Source: CAD feature listing. Evaluate the final solid. Frame: model axes, mm. Give positions to 0.01 mm unless a question says otherwise; leave off trailing zeros. Loops run counter-clockwise (first coordinate to the right, second up) from the corner with the lowest first, then second, coordinate; pieces in that order, holes last.
Autodesk Inventor part; units mm, degrees
ref_plane "YZ Plane" through (0, 0, 0) normal (1, 0, 0) x (0, 1, 0)
ref_plane "XZ Plane" through (0, 0, 0) normal (0, 1, 0) x (-1, 0, 0)
ref_plane "XY Plane" through (0, 0, 0) normal (0, 0, 1) x (1, 0, 0)
sketch "Esquisse1" plane through (0, 0, 0) normal (0, 1, 0) x (-1, 0, 0)
  line L0 (81.9588, 98.0854) -> (-168.0412, 98.0854)
  line L1 (-168.0412, 98.0854) -> (-168.0412, -201.9146)
  line L2 (-168.0412, -201.9146) -> (81.9588, -201.9146)
  line L3 (81.9588, -201.9146) -> (81.9588, 98.0854)
  point P0 (0, 0)
  dimension "d0" = 300
  dimension "d1" = 250
extrude "Extrusion1" add sketch "Esquisse1" along normal blind 5
sketch "Sketch3" plane through (0, 5, 0) normal (0, 1, 0) x (1, 0, 0)
  line L0 (81.0412, -85.0854) -> (5.0412, -85.0854)
  line L1 (5.0412, -85.0854) -> (5.0412, -17.0854)
  line L2 (81.0412, -17.0854) -> (81.0412, -85.0854)
  line L3 (-81.9588, -98.0854) -> (168.0412, -98.0854)
  line L4 (168.0412, -98.0854) -> (168.0412, 201.9146)
  line L5 (17.0412, -17.0854) -> (17.0412, 40.9146)
  line L6 (17.0412, 40.9146) -> (69.0412, 40.9146)
  line L7 (69.0412, 40.9146) -> (69.0412, -17.0854)
  line L8 (5.0412, -17.0854) -> (17.0412, -17.0854)
  line L9 (69.0412, -17.0854) -> (81.0412, -17.0854)
  line L10 (81.0412, 188.9146) -> (5.0412, 188.9146)
  line L11 (5.0412, 188.9146) -> (5.0412, 120.9146)
  line L12 (81.0412, 120.9146) -> (81.0412, 188.9146)
  line L13 (168.0412, 201.9146) -> (-81.9588, 201.9146)
  line L14 (17.0412, 120.9146) -> (17.0412, 62.9146)
  line L15 (17.0412, 62.9146) -> (69.0412, 62.9146)
  line L16 (69.0412, 62.9146) -> (69.0412, 120.9146)
  line L17 (5.0412, 120.9146) -> (17.0412, 120.9146)
  line L18 (69.0412, 120.9146) -> (81.0412, 120.9146)
  circle A0 centre (85.0412, 51.9146) radius 1.5
  line L19 (-81.9588, 201.9146) -> (-81.9588, -98.0854)
  circle A1 centre (1.0412, 51.9146) radius 1.5
  point P0 (0, 0)
  dimension "d17" = 76
  dimension "d18" = 68
  dimension "d19" = 13
  dimension "d20" = 87
  dimension "d21" = 12
  dimension "d22" = 12
  dimension "d23" = 58
  dimension "d24" = 68
  dimension "d25" = 52
  dimension "d26" = 13
  dimension "d27" = 76
  dimension "d28" = 68
  dimension "d29" = 87
  dimension "d30" = 12
  dimension "d31" = 12
  dimension "d32" = 58
  dimension "d33" = 52
  dimension "d34" = 68
  dimension "d39" = 3
  dimension "d53" = 83
  dimension "d54" = 150
  dimension "d58" = 3
  dimension "d59" = 83
  dimension "d60" = 150
extrude "Extrusion3" cut sketch "Sketch3" against normal through all contours L0 L1 L8 L5 L6 L7 L9 L2 | L12 L18 L16 L15 L14 L17 L11 L10 | A0 | A1
sketch "Sketch4" plane through (0, 5, 0) normal (0, 1, 0) x (1, 0, 0)
  circle A0 centre (1.0412, -89.0854) radius 1.5
  circle A1 centre (1.0412, -11.0854) radius 1.5
  circle A2 centre (85.0412, -89.0854) radius 1.5
  circle A3 centre (85.0412, -11.0854) radius 1.5
  circle A4 centre (1.0412, 114.9146) radius 1.5
  circle A5 centre (1.0412, 192.9146) radius 1.5
  circle A6 centre (85.0412, 192.9146) radius 1.5
  circle A7 centre (85.0412, 114.9146) radius 1.5
  point P0 (0, 0)
extrude "Extrusion4" cut sketch "Sketch4" against normal up to next
sketch "Esquisse5" plane through (0, 5, 0) normal (0, 1, 0) x (1, 0, 0)
  circle A0 centre (139.5412, -83.0854) radius 1.5
  circle A1 centre (133.0412, -83.0854) radius 1.5
  circle A2 centre (133.0412, 186.9146) radius 1.5
  circle A3 centre (139.5412, 186.9146) radius 1.5
  circle A4 centre (-41.9588, 186.9146) radius 1.5
  circle A5 centre (-48.4588, 186.9145) radius 1.4999
  circle A6 centre (-41.9588, -83.0854) radius 1.5
  circle A7 centre (85.0412, 192.9146) radius 1.5
  circle A8 centre (1.0412, 114.9146) radius 1.5
  circle A9 centre (85.0412, -89.0854) radius 1.5
  circle A10 centre (1.0412, -89.0854) radius 1.5
  circle A11 centre (1.0412, -11.0854) radius 1.5
  circle A12 centre (85.0412, -11.0854) radius 1.5
  circle A13 centre (1.0412, 192.9146) radius 1.5
  circle A14 centre (85.0412, 114.9146) radius 1.5
  line L0 (81.0412, -17.0854) -> (81.0412, -85.0854)
  line L1 (81.0412, -85.0854) -> (5.0412, -85.0854)
  line L2 (5.0412, -85.0854) -> (5.0412, -17.0854)
  line L3 (5.0412, -17.0854) -> (17.0412, -17.0854)
  line L4 (17.0412, -17.0854) -> (17.0412, 40.9146)
  line L5 (17.0412, 40.9146) -> (69.0412, 40.9146)
  line L6 (69.0412, 40.9146) -> (69.0412, -17.0854)
  line L7 (69.0412, -17.0854) -> (81.0412, -17.0854)
  circle A15 centre (85.0412, 51.9146) radius 1.5
  circle A16 centre (1.0412, 51.9146) radius 1.5
  line L8 (5.0412, 120.9146) -> (5.0412, 188.9146)
  line L9 (5.0412, 188.9146) -> (81.0412, 188.9146)
  line L10 (81.0412, 188.9146) -> (81.0412, 120.9146)
  line L11 (81.0412, 120.9146) -> (69.0412, 120.9146)
  line L12 (69.0412, 120.9146) -> (69.0412, 62.9146)
  line L13 (69.0412, 62.9146) -> (17.0412, 62.9146)
  line L14 (17.0412, 62.9146) -> (17.0412, 120.9146)
  line L15 (17.0412, 120.9146) -> (5.0412, 120.9146)
  line L16 (-81.9588, -98.0854) -> (168.0412, -98.0854)
  line L17 (168.0412, -98.0854) -> (168.0412, 201.9146)
  line L18 (168.0412, 201.9146) -> (-81.9588, 201.9146)
  line L19 (-81.9588, 201.9146) -> (-81.9588, -98.0854)
  circle A17 centre (-48.4588, -83.0854) radius 1.5
  point P0 (0, 0)
extrude "Extrusion5" cut sketch "Esquisse5" against normal up to next contours A0 | A1 | A2 | A3 | A4 | A5 | A6 | A17
sketch "Esquisse6" plane through (0, 0, 0) normal (0, -1, 0) x (1, 0, 0)
  circle A0 centre (139.0412, 63.0854) radius 1.5
  circle A1 centre (163.0412, 39.0854) radius 1.5
  circle A2 centre (139.0412, -142.9146) radius 1.5
  circle A3 centre (163.0412, -166.9146) radius 1.5
  line L0 (-81.9588, 98.0854) -> (168.0412, 98.0854)
  line L1 (168.0412, -201.9146) -> (-81.9588, -201.9146)
  line L2 (57.7912, 123.3914) -> (57.7912, -232.7016)
  line L3 (168.0412, 98.0854) -> (168.0412, -201.9146)
  circle A4 centre (-23.4588, 63.0854) radius 1.5
  circle A5 centre (-47.4588, 39.0854) radius 1.5
  circle A6 centre (-23.4588, -142.9146) radius 1.5
  circle A7 centre (-47.4588, -166.9146) radius 1.5
  point P0 (0, 0)
  dimension "d82" = 110.25
extrude "Extrusion6" cut sketch "Esquisse6" against normal up to next contours A0 | A1 | A2 | A3 | A4 | A5 | A6 | A7
sketch "Esquisse7" plane through (0, 5, 0) normal (0, 1, 0) x (1, 0, 0)
  circle A0 centre (152.0412, 161.9146) radius 1.5
  circle A1 centre (-65.9588, 51.9146) radius 1.5
  circle A2 centre (152.0412, 51.9146) radius 1.5
  circle A3 centre (152.0412, -58.0854) radius 1.5
  line L0 (-81.9588, 201.9146) -> (168.0412, 201.9146)
  line L1 (-81.9588, -98.0854) -> (-81.9588, 201.9146)
  line L2 (168.0412, -98.0854) -> (-81.9588, -98.0854)
  line L3 (168.0412, 201.9146) -> (168.0412, -98.0854)
  circle A4 centre (152.0412, 161.9146) radius 1.5
  circle A5 centre (-65.9588, 51.9146) radius 1.5
  circle A6 centre (152.0412, 51.9146) radius 1.5
  circle A7 centre (152.0412, -58.0854) radius 1.5
  line L4 (-81.9588, 201.9146) -> (168.0412, 201.9146)
  line L5 (-81.9588, -98.0854) -> (-81.9588, 201.9146)
  line L6 (168.0412, -98.0854) -> (-81.9588, -98.0854)
  line L7 (168.0412, 201.9146) -> (168.0412, -98.0854)
  circle A8 centre (152.0412, 161.9146) radius 1.5
  circle A9 centre (-65.9588, 51.9146) radius 1.5
  circle A10 centre (152.0412, 51.9146) radius 1.5
  circle A11 centre (152.0412, -58.0854) radius 1.5
  line L8 (-81.9588, 201.9146) -> (168.0412, 201.9146)
  line L9 (-81.9588, -98.0854) -> (-81.9588, 201.9146)
  line L10 (168.0412, -98.0854) -> (-81.9588, -98.0854)
  line L11 (168.0412, 201.9146) -> (168.0412, -98.0854)
  circle A12 centre (133.0412, -83.0854) radius 1.5
  circle A13 centre (-41.9588, 186.9146) radius 1.5
  circle A14 centre (133.0412, 186.9146) radius 1.5
  circle A15 centre (-48.4588, 186.9145) radius 1.4999
  circle A16 centre (139.5412, 186.9146) radius 1.5
  circle A17 centre (-41.9588, -83.0854) radius 1.5
  circle A18 centre (139.5412, -83.0854) radius 1.5
  circle A19 centre (-48.4588, -83.0854) radius 1.5
  circle A20 centre (85.0412, 192.9146) radius 1.5
  circle A21 centre (1.0412, 114.9146) radius 1.5
  circle A22 centre (85.0412, -89.0854) radius 1.5
  circle A23 centre (1.0412, -89.0854) radius 1.5
  circle A24 centre (1.0412, -11.0854) radius 1.5
  circle A25 centre (85.0412, -11.0854) radius 1.5
  circle A26 centre (1.0412, 192.9146) radius 1.5
  circle A27 centre (85.0412, 114.9146) radius 1.5
  line L12 (81.0412, -17.0854) -> (81.0412, -85.0854)
  line L13 (81.0412, -85.0854) -> (5.0412, -85.0854)
  line L14 (5.0412, -85.0854) -> (5.0412, -17.0854)
  line L15 (5.0412, -17.0854) -> (17.0412, -17.0854)
  line L16 (17.0412, -17.0854) -> (17.0412, 40.9146)
  line L17 (17.0412, 40.9146) -> (69.0412, 40.9146)
  line L18 (69.0412, 40.9146) -> (69.0412, -17.0854)
  line L19 (69.0412, -17.0854) -> (81.0412, -17.0854)
  circle A28 centre (85.0412, 51.9146) radius 1.5
  circle A29 centre (1.0412, 51.9146) radius 1.5
  line L20 (5.0412, 120.9146) -> (5.0412, 188.9146)
  line L21 (5.0412, 188.9146) -> (81.0412, 188.9146)
  line L22 (81.0412, 188.9146) -> (81.0412, 120.9146)
  line L23 (81.0412, 120.9146) -> (69.0412, 120.9146)
  line L24 (69.0412, 120.9146) -> (69.0412, 62.9146)
  line L25 (69.0412, 62.9146) -> (17.0412, 62.9146)
  line L26 (17.0412, 62.9146) -> (17.0412, 120.9146)
  line L27 (17.0412, 120.9146) -> (5.0412, 120.9146)
  line L28 (-81.9588, -98.0854) -> (168.0412, -98.0854)
  line L29 (168.0412, -98.0854) -> (168.0412, 201.9146)
  line L30 (168.0412, 201.9146) -> (-81.9588, 201.9146)
  line L31 (-81.9588, 201.9146) -> (-81.9588, -98.0854)
  circle A30 centre (100.5413, 149.4146) radius 2.0001
  circle A31 centre (120.5412, 149.4146) radius 2
  circle A32 centre (100.5412, -45.5854) radius 2
  circle A33 centre (120.5412, -45.5854) radius 2
  circle A34 centre (75.0412, 19.9146) radius 2
  circle A35 centre (11.0412, 83.9146) radius 2
  circle A36 centre (11.0412, 19.9146) radius 2
  circle A37 centre (75.0412, 83.9146) radius 2
  circle A38 centre (-61.9588, 171.9146) radius 7.5
  circle A39 centre (75.0412, 19.9146) radius 2
  circle A40 centre (11.0412, 83.9146) radius 2
  circle A41 centre (11.0412, 19.9146) radius 2
  circle A42 centre (75.0412, 83.9146) radius 2
  circle A43 centre (-61.9588, 171.9146) radius 7.5
  circle A44 centre (75.0412, 19.9146) radius 2
  circle A45 centre (11.0412, 83.9146) radius 2
  circle A46 centre (11.0412, 19.9146) radius 2
  circle A47 centre (75.0412, 83.9146) radius 2
  circle A48 centre (-61.9588, 171.9146) radius 7.5
  point P0 (0, 0)
extrude "Extrusion7" cut sketch "Esquisse7" against normal up to next contours A30 | A31 | A32 | A33
sketch "Esquisse8" plane through (0, 0, 0) normal (0, -1, 0) x (1, 0, 0)
  line L0 (-81.9588, 98.0854) -> (168.0412, 98.0854)
  line L1 (168.0412, -201.9146) -> (-81.9588, -201.9146)
  line L2 (-81.9588, 98.0854) -> (-52.9588, 98.0854)
  line L3 (-52.9588, 98.0854) -> (-52.9588, -201.9146)
  line L4 (-52.9588, -201.9146) -> (-81.9588, -201.9146)
  line L5 (-81.9588, -201.9146) -> (-81.9588, 98.0854)
  circle A0 centre (-48.4588, 83.0854) radius 1.5
  point P0 (0, 0)
  dimension "d79" = 4.5
extrude "Extrusion8" cut sketch "Esquisse8" against normal through all contours L0 L3 L1 L5
properties part number "socle-robot"
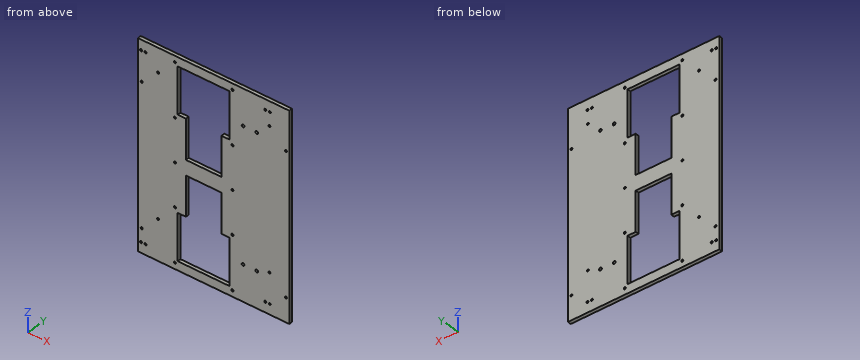
(1) Section C-C, the plane z = -31.5. Return the cut outline in (x, y).
A:
outline: (-52.96, 0) - (17.04, 0) - (17.04, 5) - (-52.96, 5) - close; (69.04, 0) - (168.04, 0) - (168.04, 5) - (69.04, 5) - close
(2) First-contact query: pin 1 (5 mm diameter, centred on x = -48.46, z = 83.09, fed in from -Y); pin 2 (2.5 mm diameter, centred on x = 85.04, z = 89.09, fed in from -Y). Flat tips, straight axial feed; report the tip coordinate or a pass-through.
A:
pin 1: stops at y = 0
pin 2: passes through
(3) Section A-A, the plane x = 23. Return the cut outline in (y, z).
A:
outline: (0, -201.91) - (5, -201.91) - (5, -188.91) - (0, -188.91) - close; (0, -62.91) - (5, -62.91) - (5, -40.91) - (0, -40.91) - close; (0, 85.09) - (5, 85.09) - (5, 98.09) - (0, 98.09) - close
(4) Ray query, line 1 along Z through (x, y) = (42, 3.1); line 2 along X through (y, z) = (1.6, -75.5); line 3 along Z through (x, y) = (77.5, 1.55). Return the intervals inside material, ascending.
A:
line 1: z = -201.91 to -188.91, -62.91 to -40.91, 85.09 to 98.09
line 2: x = -52.96 to 17.04, 69.04 to 168.04
line 3: z = -201.91 to -188.91, -120.91 to 17.09, 85.09 to 98.09
(5) Section D-D, the plane y = 1.55. Count the separate pieces of the cut face and the enclosed holes in it, then the cut area to 3 significant figures.
A:
separate pieces: 1
enclosed holes: 32
area: 49,700 mm2
(6) Section B-B, the plane z = -130. Return the cut outline in (x, y), then the cut area to 3 significant figures.
A:
outline: (-52.96, 0) - (5.04, 0) - (5.04, 5) - (-52.96, 5) - close; (81.04, 0) - (168.04, 0) - (168.04, 5) - (81.04, 5) - close
area: 725 mm2
